from build123d import *

# Parameters (mm, degrees)
PAD_DEPTH       = 40
FILLET_R        = 10
THICKNESS_T     = -5
SKETCH043_R     = 64
SKETCH043_R_2   = 23.25
POCKET007_DEPTH = 40.001
SKETCH046_R     = 26.5
POCKET009_DEPTH = 2
SKETCH045_R     = 77
POCKET010_DEPTH = 5.3
SKETCH047_R     = 82
SKETCH047_R_2   = 64
PAD028_DEPTH    = 5


with BuildPart() as part:
    # Sketch → Pad (new body)
    with BuildSketch(Plane.XY):
        with BuildLine():
            Line((-100, 490), (-100, 10))
            ThreePointArc((-100, 10), (-97.0710678119, 2.9289321881), (-90, 0))
            Line((-90, 0), (90, 0))
            ThreePointArc((90, 0), (97.0710678119, 2.9289321881), (100, 10))
            Line((100, 10), (100, 490))
            ThreePointArc((100, 490), (97.0710678119, 497.0710678119), (90, 500))
            Line((90, 500), (-90, 500))
            ThreePointArc((-90, 500), (-97.0710678119, 497.0710678119), (-100, 490))
        make_face()
    extrude(amount=-PAD_DEPTH)

    # Fillet
    fillet_edges = [part.edges().sort_by_distance(p)[0] for p in [
        (-100, 250, 0),
        (-97.071068, 2.928932, 0),
        (0, 0, 0),
        (97.071068, 2.928932, 0),
        (100, 250, 0),
        (97.071068, 497.071068, 0),
        (0, 500, 0),
        (-97.071068, 497.071068, 0),
    ]]
    fillet(fillet_edges, radius=FILLET_R)

    # Thickness
    thickness_openings = [part.faces().sort_by_distance(p)[0] for p in [
        (0, 250, -40),
    ]]
    offset(amount=THICKNESS_T, openings=thickness_openings)

    # Sketch043 → Pocket007 (cut, through all)
    with BuildSketch(Plane.XY):
        with Locations((0, 200)):
            Circle(SKETCH043_R)
        with Locations((-32.5, 250)):
            Circle(SKETCH043_R_2)
        with Locations((0, 364)):
            Circle(SKETCH043_R)
    extrude(amount=-POCKET007_DEPTH, mode=Mode.SUBTRACT)

    # Sketch046 (on Face9 of Pad) → Pocket009 (cut)
    with BuildSketch(Plane.XY):
        with Locations((-32.5, 250)):
            Circle(SKETCH046_R)
    extrude(amount=-POCKET009_DEPTH, mode=Mode.SUBTRACT)

    # Sketch045 (on Face9 of Pad) → Pocket010 (cut)
    with BuildSketch(Plane.XY):
        with Locations((0, 200)):
            Circle(SKETCH045_R)
        with Locations((0, 364)):
            Circle(SKETCH045_R)
    extrude(amount=-POCKET010_DEPTH, mode=Mode.SUBTRACT)

    # Sketch047 (on Face31 of Thickness) → Pad028 (join)
    with BuildSketch(Plane(origin=(0, 0, -5), x_dir=(-1, 0, 0), z_dir=(0, 0, -1))):
        with Locations((0, 200)):
            Circle(SKETCH047_R)
        with Locations((0, 200)):
            Circle(SKETCH047_R_2, mode=Mode.SUBTRACT)
        with Locations((0, 364)):
            Circle(SKETCH047_R)
        with Locations((0, 364)):
            Circle(SKETCH047_R_2, mode=Mode.SUBTRACT)
    extrude(amount=PAD028_DEPTH)


solid = part.part
Could you check a few things on this model? Use its own coordinates, in mm. A direction names the side the tool comes from. Give positions to 0.01 mm unless a question says otherwise; leave off trailing zeros. Order: outer loops, then holes, each group sorted by start corner. A loop starts at its lowest first (then second) coordinate and runs counter-clockwise, first axis right, second up.
Item 1: I need wall thicknesses on line 1 (X direction, y = 42.5, z = -24.5); line 2 (Y direction, x = 21, z = -25); line 3 (X direction, y = 70, z = -9). Which ranges of each line are inside material? Lowest first, please.
Item 2: If we section it at A-A, the plane y = 200: Write out the boundary of the cut face in (x, z).
Item 3: If we section it at D-D, the plane x = 52: Count the separate pieces of the cut face and the enclosed holes in it, plus the area to 3 significant figures.
Item 4: If we section it at C-C, the plane y = 65.5: Write out the boundary of the cut face in (x, z), plus the area to 3 significant figures.
Item 5: For faces 4 (the face through (11.8, 263.1, -5)), 5 (the face through (96.99, 2.85, -24.79)), 6 (the face through (-1, 5, -25)), which set-ups out of +Z, -Z, +X, -X, +Y, -Y let a thin tool reach every point of the face, with its end or its side?
Item 6: If we mould it in two halves opening along Y, with no side actions, what happens to faces 1 (the face through (-97.15, 3.01, -24.79)), 2 (the face through (96, 251, -40)), 3 (the face through (95, 247, -25))? For each: pulls with the +Y half, pulls with the -Y half, needs draft (parallel to the pull), parting line crosses it, or undercut.
Item 7: I'm going to push a flat-ended pin straight in: pin 1 (10 mm diameter, centred on x = -72, y = 305.5, fed in from +Z). Where does the tip first touch, or does it pass through?
Item 8: If we section it at B-B, the plane z = -17.5: Write out the boundary of the cut face in (x, y).
Values:
1. line 1: x = -100 to -95, 95 to 100
1. line 2: y = 0 to 5, 495 to 500
1. line 3: x = -99.95 to -94.9, 94.9 to 99.95
2. outline: (-100, -40) - (-95, -40) - (-95, -10) arc R5 cw to (-90, -5) - (-82, -5) - (-82, -10) - (-64, -10) - (-64, -5) - (-77, -5) - (-77, 0) - (-90, 0) arc R10 ccw to (-100, -10) - close; (64, -10) - (82, -10) - (82, -5) - (90, -5) arc R5 cw to (95, -10) - (95, -40) - (100, -40) - (100, -10) arc R10 ccw to (90, 0) - (77, 0) - (77, -5) - (64, -5) - close
3. separate pieces: 3
3. enclosed holes: 0
3. area: 2,200 mm2
4. outline: (-100, -40) - (-95, -40) - (-95, -10) arc R5 cw to (-90, -5) - (90, -5) arc R5 cw to (95, -10) - (95, -40) - (100, -40) - (100, -10) arc R10 ccw to (90, 0) - (-90, 0) arc R10 ccw to (-100, -10) - close
4. area: 1,320 mm2
5. face 4: +Z
5. face 5: +Z, -Z, +X, -Y
5. face 6: -Z
6. face 1: pulls with the -Y half
6. face 2: needs draft
6. face 3: undercut
7. pin 1: stops at z = 0
8. outline: (-100, 10) arc R10 ccw to (-90, 0) - (90, 0) arc R10 ccw to (100, 10) - (100, 490) arc R10 ccw to (90, 500) - (-90, 500) arc R10 ccw to (-100, 490) - close; hole (-95, 10) arc R5 ccw to (-90, 5) - (90, 5) arc R5 ccw to (95, 10) - (95, 490) arc R5 ccw to (90, 495) - (-90, 495) arc R5 ccw to (-95, 490) - close
